For this review, take the finished solid that the model builds, in its own axes (mm). Face numbers are marked on the shaded views. A direction names the side the tool comes from. Give positions to 0.01 mm unless a question says otherwise; leave off trailing zeros. Write each loop counter-clockwise with the first axis right and the second up, starting at its lowest first coordinate (ties: lowest second). Pieces come first, ordered by that corner, then holes. Notation, with made-up numbers: M 84.5,54.5 L 143.5,54.5 A33 ccw 143.5,89.5 Z; hole C 70.25,43 d4. An arc over 180 degrees is marked long. One line per item, written item: value. Start each with the question number.
Item 1: Mouldability with a two-part tool opening along X and no side actions: class the marked faces 4, 5 and 6 as released by +X, released by -X, zero draft, split by the parting line, or undercut.
Item 2: Consider section B-B, the plane x = 0. Write out the cut boundary in (y, z).
Item 3: Consider section A-A, the plane x = -14.5. Write out the cut boundary in (y, z) (3 decimals), and give its area (3 significant figures).
Item 4: Consider section C-C, the plane y = 45. Write out the cut boundary in (x, z).
Item 5: Clearance check with flat-ended pins moving along their axes: pin 1 Ø5 at (x, y) = (-2, 1) entering from -Z; pin 2 Ø2.5 at (x, y) = (-11.5, 51) entering from +Z; pin 3 Ø4 at (x, y) = (9.5, 49.5) entering from -Z; pin 4 Ø4 at (x, z) = (-1, 1.5) entering from -Y. State where each tip first meets the part, or that it passes through.
Item 6: Consider section D-D, the plane x = 15.5. Write out the cut boundary in (y, z) (3 decimals), and give its area (3 significant figures).
Item 7: To check wall thickness, follow probe 1 along Z at (x, y) = (0, 50); probe 2 along X at (y, z) = (51.6, 0); probe 3 along Z at (x, y) = (0, 34). State the ranges of each line that lie inside material, in increasing order.
Item 8: Tool access review of the marked faces 1, 2 and 3: name each direction out of +Z, -Z, +X, -X, +Y, -Y from which nothing blocks a thin tool from reaching the whole face with its end or side.
```python
from build123d import *

# Parameters (mm, degrees)
SKETCH1_R           = 19.05
BOSS_EXTRUDE1_DEPTH = 2.54
SKETCH2_R           = 12.7
BOSS_EXTRUDE2_DEPTH = 25.4
BOSS_EXTRUDE2_TAPER = 20
SKETCH3_R           = 2.54
CUT_EXTRUDE1_DEPTH  = 27.94
CUT_EXTRUDE1_TAPER  = -20
SKETCH4_R           = 19.05
SKETCH4_R_2         = 16.51
BOSS_EXTRUDE3_DEPTH = 50.8
SKETCH5_R           = 19.05
SKETCH5_R_2         = 2.54
BOSS_EXTRUDE4_DEPTH = 5.08
SKETCH6_R           = 19.05
SKETCH6_R_2         = 17.78
BOSS_EXTRUDE5_DEPTH = 5.08


with BuildPart() as part:
    # Sketch1 → Boss-Extrude1 (new body)
    with BuildSketch(Plane(origin=(0, 0, 0), x_dir=(1, 0, 0), z_dir=(0, 1, 0))):
        Circle(SKETCH1_R)
    extrude(amount=BOSS_EXTRUDE1_DEPTH)

    # Sketch2 → Boss-Extrude2 (add)
    with BuildSketch(Plane.XZ):
        Circle(SKETCH2_R)
    extrude(amount=BOSS_EXTRUDE2_DEPTH, taper=BOSS_EXTRUDE2_TAPER)

    # Sketch3 → Cut-Extrude1 (cut)
    with BuildSketch(Plane.XZ.offset(25.4)):
        Circle(SKETCH3_R)
    extrude(amount=-CUT_EXTRUDE1_DEPTH, taper=CUT_EXTRUDE1_TAPER, mode=Mode.SUBTRACT)

    # Sketch4 → Boss-Extrude3 (add)
    with BuildSketch(Plane(origin=(0, 2.54, 0), x_dir=(1, 0, 0), z_dir=(0, 1, 0))):
        Circle(SKETCH4_R)
        Circle(SKETCH4_R_2, mode=Mode.SUBTRACT)
    extrude(amount=BOSS_EXTRUDE3_DEPTH)

    # Sketch5 → Boss-Extrude4 (add)
    with BuildSketch(Plane(origin=(0, 53.34, 0), x_dir=(1, 0, 0), z_dir=(0, 1, 0))):
        Circle(SKETCH5_R)
        Circle(SKETCH5_R_2, mode=Mode.SUBTRACT)
        with BuildLine():
            Line((3.756710662, 0.635), (16.497783942, 0.635))
            ThreePointArc((16.497783942, 0.635), (0, 16.51), (-16.497783942, 0.635))
            Line((-16.497783942, 0.635), (-3.756710662, 0.635))
            ThreePointArc((-3.756710662, 0.635), (0, 3.81), (3.756710662, 0.635))
        make_face(mode=Mode.SUBTRACT)
        with BuildLine():
            Line((3.756710662, -0.635), (16.497783942, -0.635))
            ThreePointArc((16.497783942, -0.635), (0, -16.51), (-16.497783942, -0.635))
            Line((-16.497783942, -0.635), (-3.756710662, -0.635))
            ThreePointArc((-3.756710662, -0.635), (0, -3.81), (3.756710662, -0.635))
        make_face(mode=Mode.SUBTRACT)
    extrude(amount=-BOSS_EXTRUDE4_DEPTH)

    # Sketch6 → Boss-Extrude5 (add)
    with BuildSketch(Plane(origin=(0, 53.34, 0), x_dir=(1, 0, 0), z_dir=(0, 1, 0))):
        Circle(SKETCH6_R)
        Circle(SKETCH6_R_2, mode=Mode.SUBTRACT)
    extrude(amount=BOSS_EXTRUDE5_DEPTH)


solid = part.part
```
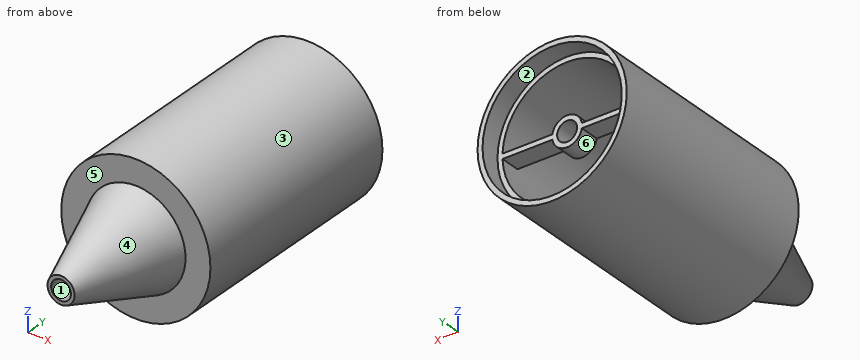
Model answer:
1. face 4: split by the parting line
1. face 5: zero draft
1. face 6: undercut
2. outline: M -25.4,-3.46 L 0,-12.7 L 0,-19.05 L 58.42,-19.05 L 58.42,-17.78 L 53.34,-17.78 L 53.34,-16.51 L 2.54,-16.51 L 2.54,-12.71 L -25.4,-2.54 Z; M -25.4,2.54 L 2.54,12.71 L 2.54,16.51 L 53.34,16.51 L 53.34,17.78 L 58.42,17.78 L 58.42,19.05 L 0,19.05 L 0,12.7 L -25.4,3.46 Z; M 48.26,-3.81 L 53.34,-3.81 L 53.34,-2.54 L 48.26,-2.54 Z; M 48.26,2.54 L 53.34,2.54 L 53.34,3.81 L 48.26,3.81 Z
3. outline: M 0,-12.355 L 58.42,-12.355 L 58.42,-10.29 L 53.34,-10.29 L 53.34,-7.895 L 2.54,-7.895 L 2.54,7.895 L 53.34,7.895 L 53.34,10.29 L 58.42,10.29 L 58.42,12.355 L 0,12.355 Z; M 48.26,-0.635 L 53.34,-0.635 L 53.34,0.635 L 48.26,0.635 Z
3. area: 543 mm2
4. outline: C 0,0 d38.1; hole C 0,0 d33.02
5. pin 1: stops at z = -19.05
5. pin 2: stops at z = 16.06
5. pin 3: stops at z = -17.51
5. pin 4: stops at y = -25.4
6. outline: M 0,-11.075 L 58.42,-11.075 L 58.42,-8.711 L 53.34,-8.711 L 53.34,-5.686 L 2.54,-5.686 L 2.54,5.686 L 53.34,5.686 L 53.34,8.711 L 58.42,8.711 L 58.42,11.075 L 0,11.075 Z; M 48.26,-0.635 L 53.34,-0.635 L 53.34,0.635 L 48.26,0.635 Z
6. area: 634 mm2
7. probe 1: z = -19.05 to -16.51, -3.81 to -2.54, 2.54 to 3.81, 16.51 to 19.05
7. probe 2: x = -19.05 to -2.54, 2.54 to 19.05
7. probe 3: z = -19.05 to -16.51, 16.51 to 19.05
8. face 1: none
8. face 2: +Y
8. face 3: +Y, -Y
